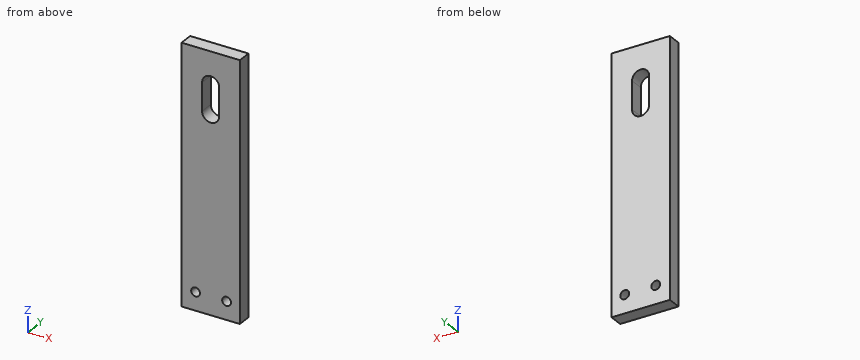
from build123d import *

# Parameters (mm, degrees)
SKETCH1_W           = 12.6
SKETCH1_H           = 55
BOSS_EXTRUDE1_DEPTH = 3
SKETCH2_R           = 0.95
CUT_EXTRUDE1_DEPTH  = 57.504513094


with BuildPart() as part:
    # Sketch1 → Boss-Extrude1 (new body)
    with BuildSketch(Plane(origin=(0, 0, 0), x_dir=(1, 0, 0), z_dir=(0, 1, 0))):
        with Locations((-6.3, 27.5)):
            Rectangle(SKETCH1_W, SKETCH1_H)
        with BuildLine():
            Line((-8.15, 7), (-8.15, 13))
            ThreePointArc((-8.15, 13), (-6.3, 14.85), (-4.45, 13))
            Line((-4.45, 13), (-4.45, 7))
            ThreePointArc((-4.45, 7), (-6.3, 5.15), (-8.15, 7))
        make_face(mode=Mode.SUBTRACT)
    extrude(amount=BOSS_EXTRUDE1_DEPTH)

    # Sketch2 → Cut-Extrude1 (cut, through all)
    with BuildSketch(Plane.XZ):
        with Locations(Location((-2.86, -51.1, 0), (0, 0, 270))):
            Circle(SKETCH2_R)
        with Locations(Location((-9.56, -51.1, 0), (0, 0, 270))):
            Circle(SKETCH2_R)
    extrude(amount=-CUT_EXTRUDE1_DEPTH, mode=Mode.SUBTRACT)


solid = part.part
Read the model definition and answer for the solid it produces. Units are mm, in the model's axes. Coordinates: 2 decimals unless noted, no trailing zeros. Write each loop counter-clockwise with the first axis right and the second up, starting at its lowest first coordinate (ties: lowest second). Pieces come first, ordered by that corner, then holes. Notation, with made-up numbers: M 76.5,1 L 100.5,1 A33 ccw 100.5,30 Z; hole C -0.5,60 d8. An arc over 180 degrees is marked long. Use a Markdown table: item, result.
Q1. The part is cut by section A-A, the plane x = -9.56. Write down the section's boundary in (y, z).
Answer block:
| item | result |
|---|---|
| outline | M 0,-55 L 3,-55 L 3,-52.05 L 0,-52.05 Z; M 0,-50.15 L 3,-50.15 L 3,0 L 0,0 Z |
Q2. The part is cut by section B-B, the plane z = -51.1. Write down the section's boundary in (x, y), then the cut area to 3 significant figures.
Answer block:
| item | result |
|---|---|
| outline | M -12.6,0 L -10.51,0 L -10.51,3 L -12.6,3 Z; M -8.61,0 L -3.81,0 L -3.81,3 L -8.61,3 Z; M -1.91,0 L 0,0 L 0,3 L -1.91,3 Z |
| area | 26.4 mm2 |
Q3. The part is cut by section D-D, the plane x = -6.3. Write down the section's boundary in (y, z), then the cut area to 3 significant figures.
Answer block:
| item | result |
|---|---|
| outline | M 0,-55 L 3,-55 L 3,-14.85 L 0,-14.85 Z; M 0,-5.15 L 3,-5.15 L 3,0 L 0,0 Z |
| area | 136 mm2 |
Q4. Straight lines are drawn through the part: L1, parallel to X at y = 1.65, z = -51.1; L2, parallel to Z at x = -9.5, y = 1.3; L3, parallel to Z at x = -3.5, y = 1.6. For each, find the intervals that lie inside material, in ascending order. Write a range as [from, to].
Answer block:
| item | result |
|---|---|
| L1 | x = [-12.6, -10.51], [-8.61, -3.81], [-1.91, 0] |
| L2 | z = [-55, -52.05], [-50.15, 0] |
| L3 | z = [-55, -51.8], [-50.4, 0] |
Q5. The part is cut by section C-C, the plane y = 0.45. Write down the section's boundary in (x, z), then the cut area to 3 significant figures.
Answer block:
| item | result |
|---|---|
| outline | M -12.6,-55 L 0,-55 L 0,0 L -12.6,0 Z; hole C -9.56,-51.1 d1.9; hole M -8.15,-13 A1.85 ccw -4.45,-13 L -4.45,-7 A1.85 ccw -8.15,-7 Z; hole C -2.86,-51.1 d1.9 |
| area | 654 mm2 |
